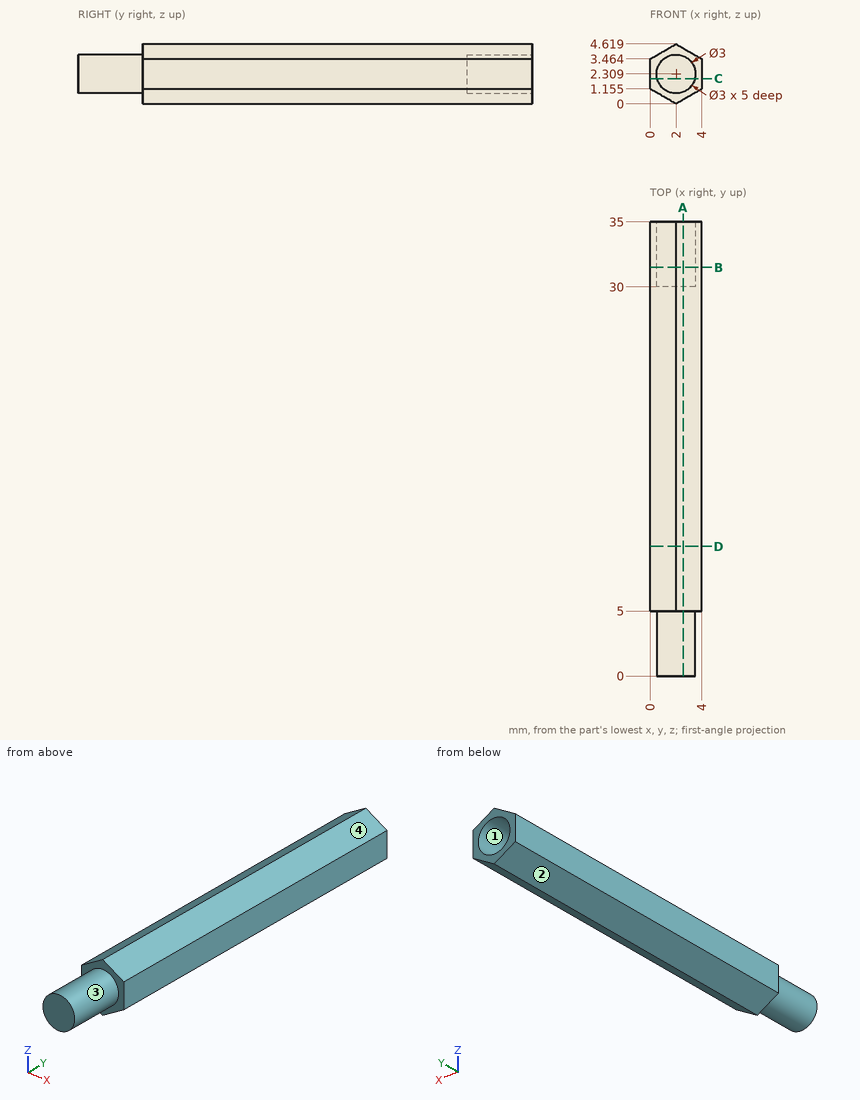
Job drawing, mm, ordinate dimensions from the low corner. One solid piece. Coordinates: 2 decimals unless noted, no trailing zeros. Write each loop counter-clockwise with the first axis right and the second up, starting at its lowest first coordinate (ties: lowest second). Pieces come first, ordered by that corner, then holes. Notation, with made-up numbers: (57, 47) - (96, 47) arc R12 cw to (96, 61) - close; hole circle Ø2 at (80, 57). An arc over 180 degrees is marked (long way). Use a Markdown table: item, result. Add a question column.
Item 1: Drill centre lines: L1, parallel to Y at x = 3.15, z = 2.7; L2, parallel to Y at x = 1.2, z = 4.05; L3, parallel to Z at x = 2.4, y = 30.5 (1 decimal). Where is each one in solid material? Low to high. Write a range as from..to.
Item 2: Band-saw the part on A-A, the plane x = 2.55. Give the cut face in (y, z) (1 decimal).
Item 3: Mould opens along X. For the marked faces 1, 2, 3 and 4 say: pulls with the +X half, pulls with the -X half, needs draft (parallel to the pull), parting line crosses it, or undercut.
Item 4: Band-saw the part on D-D, the plane y = 10. Give the cut face in (x, z) (1 decimal).
Item 5: Band-saw the part on B-B, the plane y = 31.5. Give the cut face in (x, z) (1 decimal).
Item 6: Flat gauge pins, fed straight in: pin 1 (2 mm diameter, centred on x = 1.5, z = 2, fed in from -Y); pin 2 (1.5 mm diameter, centred on x = 2, z = 2.5, fed in from +Y). Where does each tip first touch, or does it go through?
Item 7: Band-saw the part on C-C, the plane z = 1.95. Give the cut face in (x, y), and give its area (3 significant figures).
Numbers:
| question | item | result |
|---|---|---|
| 1 | L1 | 0..30 |
| 1 | L2 | 5..35 |
| 1 | L3 | 0.2..0.9, 3.8..4.4 |
| 2 | outline | (0, 0.9) - (5, 0.9) - (5, 0.3) - (35, 0.3) - (35, 0.9) - (30, 0.9) - (30, 3.7) - (35, 3.7) - (35, 4.3) - (5, 4.3) - (5, 3.7) - (0, 3.7) - close |
| 3 | face 1 | undercut |
| 3 | face 2 | pulls with the -X half |
| 3 | face 3 | parting line crosses it |
| 3 | face 4 | pulls with the +X half |
| 4 | outline | (0, 1.2) - (2, 0) - (4, 1.2) - (4, 3.5) - (2, 4.6) - (0, 3.5) - close |
| 5 | outline | (0, 1.2) - (2, 0) - (4, 1.2) - (4, 3.5) - (2, 4.6) - (0, 3.5) - close; hole circle Ø3 at (2, 2.3) |
| 6 | pin 1 | y = 0 |
| 6 | pin 2 | y = 30 |
| 7 | outline | (0, 5) - (0.54, 5) - (0.54, 0) - (3.46, 0) - (3.46, 5) - (4, 5) - (4, 35) - (3.46, 35) - (3.46, 30) - (0.54, 30) - (0.54, 35) - (0, 35) - close |
| 7 | area | 120 mm2 |
